```python
from build123d import *

# Parameters (mm, degrees)
F0_W     = 80
F0_H     = 80
F0_W_2   = 30
F0_H_2   = 6
F1_DEPTH = 8
F2_W     = 70
F2_H     = 5
F3_DEPTH = 30
F4_R     = 3
F5_DEPTH = 2


with BuildPart() as f1:
    # F0 (on Top) → F1 (new body)
    with BuildSketch(Plane.XY):
        with Locations((-40, 40)):
            Rectangle(F0_W, F0_H)
        with Locations((-40, 40)):
            Rectangle(F0_W_2, F0_H_2, mode=Mode.SUBTRACT)
    extrude(amount=F1_DEPTH)

    # F2 (on face) → F3 (join)
    with BuildSketch(Plane.XY.offset(8)):
        Polygon((-80, 80), (-80, 0), (-75, 0), (-75, 5), (-75, 80), align=None)
        with Locations((-40, 2.5)):
            Rectangle(F2_W, F2_H)
        Polygon((-5, 5), (-5, 0), (0, 0), (0, 80), (-5, 80), align=None)
    extrude(amount=F3_DEPTH)

    # F4 (on face) → F5 (join)
    with BuildSketch(Plane(origin=(0, 0, 0), x_dir=(1, 0, 0), z_dir=(0, 0, -1))):
        with Locations((-67.5, -40)):
            Circle(F4_R)
        with Locations((-12.5, -40)):
            Circle(F4_R)
    extrude(amount=F5_DEPTH)


solid = f1.part
```
Build history of the part. All positions in model axes, mm. A direction names the side the tool comes from. Round coordinates to 2 decimals unless told otherwise and drop trailing zeros. Write each loop counter-clockwise with the first axis right and the second up, starting at its lowest first coordinate (ties: lowest second). Pieces come first, ordered by that corner, then holes. Notation, with made-up numbers: (-35, 83) - (-16, 83) arc R22 cw to (-16, 106) - close; hole circle Ø11 at (79.5, 51). An arc over 180 degrees is marked (long way). Write each question's results on one line, items separated by ' | '. Start each with the question number.
Item 1: Saw through at A-A (x = -37.5). Write the cut outline in (y, z), and give its area (3 significant figures).
Item 2: Saw through at B-B (y = 40). Write the cut outline in (x, z).
Item 3: Which spindle directions (+Z, -Z, +X, -X, +Y, -Y) get a long thin tool onto all of the face, cutting with end or side? Do faces 5 (the face through (-14.71, 37.97, -0.99)), 6 (the face through (-40, 5, 23)), 7 (the face through (-68, 40, -2)), 8 (the face through (0, 39, 19)), 9 (the face through (-40, 37, 4)). Say none if no direction does.
Item 4: Drop flat-ended pins along their axis: P1, Ø1.5, axis at x = -69, y = 13.5, coming from the +Z side; P2, Ø15, axis at x = -40.5, z = 25.5, coming from the +Y side; P3, Ø12, axis at x = -28.5, y = 38.5, coming from the -Z side. Give the stop position or say it passes through.
Item 5: Saw through at D-D (x = -67.5). Write the cut outline in (y, z).
Item 6: Mould opens along X. For faces 1 (the face through (-80, 41, 19)), 2 (the face through (-13, 40, -2)), 3 (the face through (-40, 35, 8)), 4 (the face through (-25, 40, 4)) say: pulls with the +X half, pulls with the -X half, needs draft (parallel to the pull), parting line crosses it, or undercut.
Item 7: Wall check: L1, parallel to X at y = 70.5, z = 32; L2, parallel to Y at x = -32, z = 0.5; L3, parallel to Z at x = -45.5, y = 4. Give the ranges that are in metal, low to high. Write a range as [from, to].
Item 8: Saw through at C-C (z = 2.5). Write the cut outline in (x, y), and give its area (3 significant figures).
Results are:
1) outline: (0, 0) - (37, 0) - (37, 8) - (5, 8) - (5, 38) - (0, 38) - close; (43, 0) - (80, 0) - (80, 8) - (43, 8) - close | area: 742 mm²
2) outline: (-80, 0) - (-70.5, 0) - (-70.5, -2) - (-64.5, -2) - (-64.5, 0) - (-55, 0) - (-55, 8) - (-75, 8) - (-75, 38) - (-80, 38) - close; (-25, 0) - (-15.5, 0) - (-15.5, -2) - (-9.5, -2) - (-9.5, 0) - (0, 0) - (0, 38) - (-5, 38) - (-5, 8) - (-25, 8) - close
3) face 5: -Z | face 6: +Z, +Y | face 7: -Z, +X, -X, +Y, -Y | face 8: +Z, -Z, +X, +Y, -Y | face 9: +Z, -Z
4) P1: stops at z = 8 | P2: stops at y = 5 | P3: stops at z = 0
5) outline: (0, 0) - (37, 0) - (37, -2) - (43, -2) - (43, 0) - (80, 0) - (80, 8) - (5, 8) - (5, 38) - (0, 38) - close
6) face 1: pulls with the -X half | face 2: needs draft | face 3: undercut | face 4: undercut
7) L1: x = [-80, -75], [-5, 0] | L2: y = [0, 37], [43, 80] | L3: z = [0, 38]
8) outline: (-80, 0) - (0, 0) - (0, 80) - (-80, 80) - close; hole (-55, 37) - (-25, 37) - (-25, 43) - (-55, 43) - close | area: 6,220 mm²
